```python
from build123d import *

# Parameters (mm, degrees)
RESSALTO_EXTRUS_O1_DEPTH = 3


with BuildPart() as part:
    # Esboço1 → Ressalto-extrusão1 (new body)
    with BuildSketch(Plane.XY):
        with BuildLine():
            Line((-5, 15), (-5, 30))
            ThreePointArc((-5, 30), (0, 35), (5, 30))
            Line((5, 30), (5, 28))
            Line((5, 28), (15, 28))
            Line((15, 28), (15, 29))
            ThreePointArc((15, 29), (20, 34), (25, 29))
            Line((25, 29), (25, -1))
            ThreePointArc((25, -1), (20, -6), (15, -1))
            Line((15, -1), (15, 20))
            Line((15, 20), (5, 20))
            Line((5, 20), (5, 15))
            ThreePointArc((5, 15), (0, 10), (-5, 15))
        make_face()
        with BuildLine():
            Line((2, 30), (2, 15))
            ThreePointArc((2, 15), (0, 13), (-2, 15))
            Line((-2, 15), (-2, 30))
            ThreePointArc((-2, 30), (0, 32), (2, 30))
        make_face(mode=Mode.SUBTRACT)
        with BuildLine():
            Line((22, 29), (22, -1))
            ThreePointArc((22, -1), (20, -3), (18, -1))
            Line((18, -1), (18, 29))
            ThreePointArc((18, 29), (20, 31), (22, 29))
        make_face(mode=Mode.SUBTRACT)
    extrude(amount=RESSALTO_EXTRUS_O1_DEPTH)


solid = part.part
```
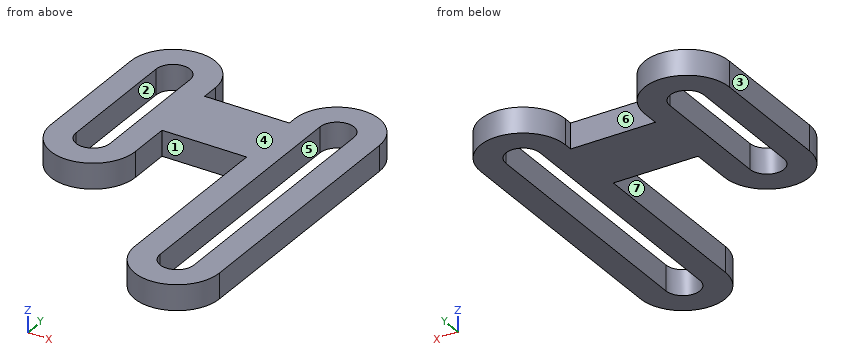
Design review of the part built by this model. Coordinates are the model's own, in mm. Face numbers are marked on the shaded views. A direction names the side the tool comes from. Give positions to 0.01 mm unless a question says otherwise; leave off trailing zeros. Order: outer loops, then holes, each group sorted by start corner. A loop starts at its lowest first (then second) coordinate and runs counter-clockwise, first axis right, second up. Notation, with made-up numbers: (69, -21) - (79, -21) arc R18 ccw to (79, -5) - close; hole circle Ø5 at (6, 51). An arc over 180 degrees is marked (long way). Use a Markdown table: item, result. Add a question column.
(1) Mouldability with a two-part tool opening along Y and no side actions: class the marked faces 1, 2 and 3 as +Y half, -Y half, draft (parallel to the pull), parting line (faces both ways), or undercut.
(2) Wall thickness on probe 1 along X at (y, z) = (18, 1.2); probe 2 along X at (y, z) = (23.5, 0.3); probe 3 along X at (y, z) = (4.5, 0.6): over which ranges is each line inside the solid? List them lowest first. Write a range as [from, to].
(3) Clearance check with flat-ended pins moving along their axes: P1, Ø1.5, axis at x = 12, z = 1.5, coming from the +Y side; P2, Ø1.5, axis at y = 12.5, z = 1, coming from the -X side. State where each tip first meets the part, or that it passes through.
(4) Machinability: for the marked faces 4, 5, 6 and 7, which of the approach directions +Z, -Z, +X, -X, +Y, -Y give a long, thin tool a straight path to every point of the face, cutting with its end or side? Answer none if there is none.
(5) Add section B-B on y = 16.5. Give the boundary of the cut face in (x, z), then the cut area to 3 significant figures.
(6) Add section C-C on y = 3.5. Give the boundary of the cut face in (x, z).
(7) Add section A-A on x = 20. Give the boundary of the cut face in (y, z), then the cut area to 3 significant figures.
(8) Add section D-D on z = 2.3. Give the boundary of the cut face in (x, y).
Report:
| question | item | result |
|---|---|---|
| 1 | face 1 | -Y half |
| 1 | face 2 | undercut |
| 1 | face 3 | draft |
| 2 | probe 1 | x = [-5, -2], [2, 5], [15, 18], [22, 25] |
| 2 | probe 2 | x = [-5, -2], [2, 18], [22, 25] |
| 2 | probe 3 | x = [15, 18], [22, 25] |
| 3 | P1 | stops at y = 28 |
| 3 | P2 | stops at x = -4.68 |
| 4 | face 4 | +Z, +X, -X, +Y, -Y |
| 4 | face 5 | +Z, -Z |
| 4 | face 6 | +Z, -Z, +Y |
| 4 | face 7 | +Z, -Z, -Y |
| 5 | outline | (-5, 0) - (-2, 0) - (-2, 3) - (-5, 3) - close; (2, 0) - (5, 0) - (5, 3) - (2, 3) - close; (15, 0) - (18, 0) - (18, 3) - (15, 3) - close; (22, 0) - (25, 0) - (25, 3) - (22, 3) - close |
| 5 | area | 36.0 mm² |
| 6 | outline | (15, 0) - (18, 0) - (18, 3) - (15, 3) - close; (22, 0) - (25, 0) - (25, 3) - (22, 3) - close |
| 7 | outline | (-6, 0) - (-3, 0) - (-3, 3) - (-6, 3) - close; (31, 0) - (34, 0) - (34, 3) - (31, 3) - close |
| 7 | area | 18.0 mm² |
| 8 | outline | (-5, 15) arc R5 ccw to (5, 15) - (5, 20) - (15, 20) - (15, -1) arc R5 ccw to (25, -1) - (25, 29) arc R5 ccw to (15, 29) - (15, 28) - (5, 28) - (5, 30) arc R5 ccw to (-5, 30) - close; hole (-2, 15) arc R2 ccw to (2, 15) - (2, 30) arc R2 ccw to (-2, 30) - close; hole (18, -1) arc R2 ccw to (22, -1) - (22, 29) arc R2 ccw to (18, 29) - close |
